```python
from build123d import *

# Parameters (mm, degrees)
F0_R     = 6.325
F2_DEPTH = 1.79
F1_R     = 4.775
F3_DEPTH = 7.39
F5_D     = 6.35


with BuildPart() as f2:
    # F0 (on Top) → F2 (new body)
    with BuildSketch(Plane.XY):
        Circle(F0_R)
    extrude(amount=F2_DEPTH)

    # F1 (on Top) → F3 (join)
    with BuildSketch(Plane.XY):
        Circle(F1_R)
    extrude(amount=F3_DEPTH)

    # F5 (through all)
    with Locations(Plane(origin=(0, 0, 0), x_dir=(1, 0, 0), z_dir=(0, 0, -1))):
        with Locations((0, 0)):
            Hole(F5_D / 2)


solid = f2.part
```
Input: part model. Units: mm. Frame: model coordinates. Coordinates: 2 decimals unless noted, no trailing zeros. Loops run counter-clockwise (first coordinate to the right, second up) from the corner with the lowest first, then second, coordinate; pieces in that order, holes last. Notation, with made-up numbers: M 57,32.5 L 77,32.5 A17 cw 77,44.5 Z; hole C 14,-4 d10. An arc over 180 degrees is marked long. Answer in a Markdown table with one row per item.
1. Section C-C, the plane z = 6.75. Output: boundary loops of the cut face in (x, y) (3 decimals), then the cut area to 3 significant figures.
Response:
| item | result |
|---|---|
| outline | C 0,0 d9.55; hole C 0,0 d6.35 |
| area | 40.0 mm2 |
2. Draft query along Y for faces 1 (the cylindrical face through (-3.789, -2.906, 4.551)), 2 (the cylindrical face through (0.69, 3.1, 3.75)), 3 (the flat face through (1, 5, 1.79)). Return one class per face: pulls with the +Y half, pulls with the -Y half, needs draft (parallel to the pull), parting line crosses it, or undercut.
Response:
| item | result |
|---|---|
| face 1 | parting line crosses it |
| face 2 | undercut |
| face 3 | needs draft |
3. Section D-D, the plane y = -4.5. Output: boundary loops of the cut face in (x, z).
Response:
| item | result |
|---|---|
| outline | M -4.44,0 L 4.44,0 L 4.44,1.79 L 1.6,1.79 L 1.6,7.39 L -1.6,7.39 L -1.6,1.79 L -4.44,1.79 Z |
4. Material intervals for line 1 (Y direction, x = 0, z = 1.5) (3 decimals); line 2 (Y direction, x = 0, z = 5.75) (3 decimals); line 3 (Z direction, x = 1, y = -5.75), sorted ascending.
Response:
| item | result |
|---|---|
| line 1 | y = -6.325 to -3.175, 3.175 to 6.325 |
| line 2 | y = -4.775 to -3.175, 3.175 to 4.775 |
| line 3 | z = 0 to 1.79 |
5. First-contact query: pin 1 (4 mm diameter, centred on x = 1.5, y = -4, fed in from -Z); pin 2 (2 mm diameter, centred on y = -2.5, z = 1.5, fed in from +X). Flat tips, straight axial feed; report the tip coordinate or a pass-through.
Response:
| item | result |
|---|---|
| pin 1 | stops at z = 0 |
| pin 2 | stops at x = 6.14 |
6. Section A-A, the plane x = 0. Output: boundary loops of the cut face in (y, z) (3 decimals), then the cut area to 3 significant figures.
Response:
| item | result |
|---|---|
| outline | M -6.325,0 L -3.175,0 L -3.175,7.39 L -4.775,7.39 L -4.775,1.79 L -6.325,1.79 Z; M 3.175,0 L 6.325,0 L 6.325,1.79 L 4.775,1.79 L 4.775,7.39 L 3.175,7.39 Z |
| area | 29.2 mm2 |
